Input: part model. Units: mm. Frame: model coordinates. Face numbers are marked on the shaded views. A direction names the side the tool comes from. Give positions to 0.01 mm unless a question says otherwise; leave off trailing zeros. Loops run counter-clockwise (first coordinate to the right, second up) from the corner with the lowest first, then second, coordinate; pieces in that order, holes last. Notation, with made-up numbers: (-15, 34.5) -> (42, 34.5) arc R18 cw to (42, 49.5) -> close; hole circle Ø4 at (50, -11). An arc over 180 degrees is marked (long way). Answer as a JSON object with one key per item and string values.
```python
from build123d import *

# Parameters (mm, degrees)
SKETCH_1_W          = 1.2
SKETCH_1_H          = 4
SKETCH_2_R          = 2
EXTRUDE_1_DEPTH     = 8
CUT_EXTRUDE_1_DEPTH = 1.2


with BuildPart() as part:
    # 草图1 → 旋转1 (revolve)
    with BuildSketch(Plane.XY):
        with Locations((-0.6, 2)):
            Rectangle(SKETCH_1_W, SKETCH_1_H)
    revolve(axis=Axis((0, 0, 0), (-1, 0, 0)))

    # 草图2 → 凸台-拉伸1 (add)
    with BuildSketch(Plane.ZY.offset(1.2)):
        with Locations(Location((0, 0, 0), (0, 0, 270))):
            Circle(SKETCH_2_R)
    extrude(amount=EXTRUDE_1_DEPTH)

    # 草图3 → 切除-拉伸1 (cut)
    with BuildSketch(Plane(origin=(0, 0, 0), x_dir=(0, 0, -1), z_dir=(1, 0, 0))):
        Polygon((0.75, 1.299038106), (-0.75, 1.299038106), (-1.5, 0), (-0.75, -1.299038106), (0.75, -1.299038106), (1.5, 0), align=None)
    extrude(amount=-CUT_EXTRUDE_1_DEPTH, mode=Mode.SUBTRACT)


solid = part.part
```
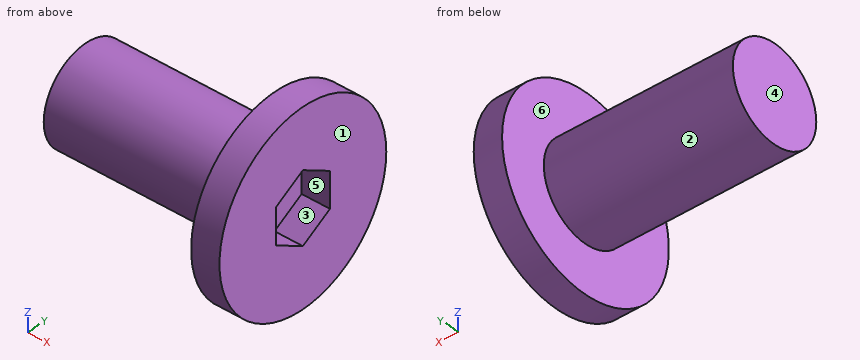
Q1. Ray query, line 1 along X through (y, z) = (1.5, -3); line 2 along X through (y, z) = (0.25, -0.5); line 3 along Z through (x, y) = (-1, 3). Return the intervals inside material, ascending.
Evaluation:
{"line 1": "x = -1.2 to 0", "line 2": "x = -9.2 to -1.2", "line 3": "z = -2.65 to 2.65"}
Q2. Section B-B, the plane z = 0. Return the cut outline in (x, y), then the cut area to 3 significant figures.
Evaluation:
{"outline": "(-9.2, -2) -> (-1.2, -2) -> (-1.2, -4) -> (0, -4) -> (0, -1.3) -> (-1.2, -1.3) -> (-1.2, 1.3) -> (0, 1.3) -> (0, 4) -> (-1.2, 4) -> (-1.2, 2) -> (-9.2, 2) -> close", "area": "38.5 mm2"}
Q3. Section D-D, the plane y = 3. Return the cut outline in (x, z), then the cut area to 3 significant figures.
Evaluation:
{"outline": "(-1.2, -2.65) -> (0, -2.65) -> (0, 2.65) -> (-1.2, 2.65) -> close", "area": "6.35 mm2"}
Q4. Access query for the marked faces 4, 5 and 6. Directions: +Z, -Z, +X, -X, +Y, -Y. A direction counts if a zero-diameter tool reaches every point of the face in a straight line with its end or side. Return the directions, or none.
Evaluation:
{"face 4": "+Z, -Z, -X, +Y, -Y", "face 5": "+X", "face 6": "-X"}
Q5. Pin query (flat end, axial travel): pin 1 (2 mm diameter, centred on x = -6, z = 2, fed in from -Y); pin 2 (3 mm diameter, centred on x = -3.5, z = -2, fed in from +Y); pin 3 (1.3 mm diameter, centred on x = -0.5, z = 0.5, fed in from +Y); pin 4 (1.5 mm diameter, centred on y = 0, z = 0.5, fed in from +X). Return the tip coordinate at first contact, or that it passes through.
Evaluation:
{"pin 1": "stops at y = -1.73", "pin 2": "stops at y = 1.94", "pin 3": "stops at y = 4", "pin 4": "stops at x = -1.2"}
Q6. Draft query along Z for the marked faces 1, 2 and 3. Return one class per face: +Z half, -Z half, draft (parallel to the pull), parting line (faces both ways), or undercut.
Evaluation:
{"face 1": "draft", "face 2": "parting line", "face 3": "undercut"}
Q7. Section C-C, the plane x = -2. Return the cut outline in (y, z), then the cut area to 3 significant figures.
Evaluation:
{"outline": "circle Ø4 at (0, 0)", "area": "12.6 mm2"}
Q8. Section A-A, the plane x = -1. Return the cut outline in (y, z).
Evaluation:
{"outline": "circle Ø8 at (0, 0); hole (-1.3, -0.75) -> (0, -1.5) -> (1.3, -0.75) -> (1.3, 0.75) -> (0, 1.5) -> (-1.3, 0.75) -> close"}
